The model under review builds one solid part; all positions refer to its coordinate system, in mm. Face numbers are marked on the shaded views. A direction names the side the tool comes from. Give positions to 0.01 mm unless a question says otherwise; leave off trailing zeros. Loops run counter-clockwise (first coordinate to the right, second up) from the corner with the lowest first, then second, coordinate; pieces in that order, holes last. Notation, with made-up numbers: (-16, 59) -> (-12, 59) arc R16 ccw to (-12, 78) -> close; hole circle Ø10 at (42.25, 31). An arc over 180 degrees is marked (long way). Write each question's results on one line, items separated by ' | '. Start each with the question number.
Q1. We need section D-D (x = -2.5). Write out the cut boundary in (y, z), plus the area to 3 significant figures.
Q2. Wall thickness on L1, parallel to X at y = -40.5, z = 3.75; L2, parallel to X at y = -39, z = 4.25; L3, parallel to Y at x = 0, z = 3.5: over which ranges is each line inside the solid? List them lowest first. Write a range as [from, to].
Q3. We need section B-B (x = 34.5). Write out the cut boundary in (y, z), plus the area to 3 significant figures.
Q4. We need section C-C (y = 0). Write out the cut boundary in (x, z).
Q5. Machinability: for the marked faces 1 and 2, which of the approach directions +Z, -Z, +X, -X, +Y, -Y give a long, thin tool a straight path to every point of the face, cutting with its end or side? Answer none if there is none.
Q6. Insertion check: pin 1 Ø1.5 at (y, z) = (-27, 3.5) entering from +X. The pin has a flat end and moves straight along its axis. Give the tip position at first contact, or say it passes through.
Q7. We need section A-A (z = 2.25). Give the number of separate pieces and of enclosed holes in the cut face, plus the area to 3 significant figures.
Q8. Mouldability with a two-part tool opening along Y and no side actions: class the marked faces 3, 4 and 5 as released by +Y, released by -Y, zero draft, split by the parting line, or undercut.
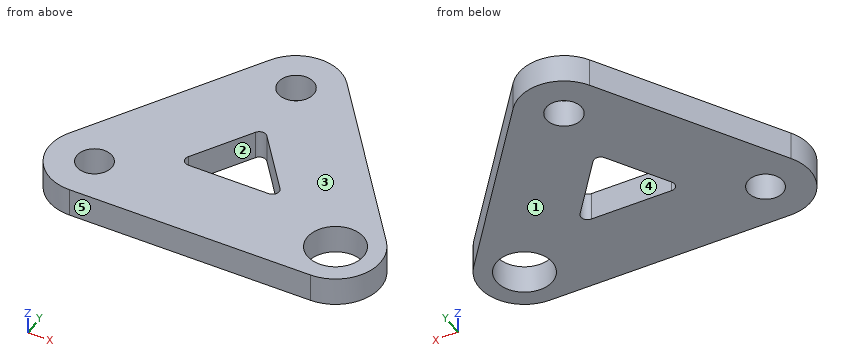
from build123d import *

# Parameters (mm, degrees)
SKETCH1_R           = 10
SKETCH1_R_2         = 3.875
SKETCH1_R_3         = 3.9375
SKETCH1_R_4         = 6.223
BOSS_EXTRUDE1_DEPTH = 6.35
FILLET1_R           = 1.5


with BuildPart() as part:
    # Sketch1 → Boss-Extrude1 (new body)
    # profile 1 of 4: a face of its own
    with BuildSketch(Plane.XY):
        with BuildLine():
            Line((-8.593850937, 5.113289165), (-31.697797638, -33.717269329))
            ThreePointArc((-31.697797638, -33.717269329), (-20.452391437, -29.188501934), (-13.103946701, -38.830558493))
            ThreePointArc((-13.103946701, -38.830558493), (-16.032878889, -45.901626305), (-23.103946701, -48.830558493))
            Line((-23.103946701, -48.830558493), (30.579912659, -48.830558493))
            ThreePointArc((30.579912659, -48.830558493), (21.583526758, -34.464205241), (38.436192426, -32.643566638))
            Line((38.436192426, -32.643566638), (7.856279768, 6.186991855))
            ThreePointArc((7.856279768, 6.186991855), (9.44888347, 3.273927483), (10, 0))
            ThreePointArc((10, 0), (-2.651555264, -9.642056559), (-8.593850937, 5.113289165))
        make_face()
        Polygon((-9.254840748, -30.955558493), (0.905857228, -13.878581033), (14.354349844, -30.955558493), align=None, mode=Mode.SUBTRACT)
    # profile 2 of 4: a face of its own
    with BuildSketch(Plane.XY):
        with Locations((-23.103946701, -38.830558493)):
            Circle(SKETCH1_R)
        with Locations((-23.103946701, -38.830558493)):
            Circle(SKETCH1_R_2, mode=Mode.SUBTRACT)
    # profile 3 of 4: a face of its own
    with BuildSketch(Plane.XY):
        Circle(SKETCH1_R)
        Circle(SKETCH1_R_3, mode=Mode.SUBTRACT)
    # profile 4 of 4: a face of its own
    with BuildSketch(Plane.XY):
        with Locations((30.579912659, -38.830558493)):
            Circle(SKETCH1_R)
        with Locations((30.579912659, -38.830558493)):
            Circle(SKETCH1_R_4, mode=Mode.SUBTRACT)
    extrude(amount=BOSS_EXTRUDE1_DEPTH)

    # Fillet1
    fillet1_edges = [part.edges().sort_by_distance(p)[0] for p in [
        (0.905857228, -13.878581033, 3.175),
        (-9.254840748, -30.955558493, 3.175),
        (14.354349844, -30.955558493, 3.175),
    ]]
    fillet(fillet1_edges, radius=FILLET1_R)


solid = part.part
Output:
1) outline: (-48.83, 0) -> (-30.96, 0) -> (-30.96, 6.35) -> (-48.83, 6.35) -> close; (-19.6, 0) -> (-3.04, 0) -> (-3.04, 6.35) -> (-19.6, 6.35) -> close; (3.04, 0) -> (9.68, 0) -> (9.68, 6.35) -> (3.04, 6.35) -> close | area: 261 mm2
2) L1: [-32.96, -26.6], [-19.61, 24.59], [36.57, 40.44] | L2: [-33.1, -26.98], [-19.23, 24.36], [36.8, 40.58] | L3: [-48.83, -30.96], [-15.48, -3.94], [3.94, 10]
3) outline: (-48.03, 0) -> (-43.66, 0) -> (-43.66, 6.35) -> (-48.03, 6.35) -> close; (-34, 0) -> (-27.65, 0) -> (-27.65, 6.35) -> (-34, 6.35) -> close | area: 68.1 mm2
4) outline: (-11.64, 0) -> (-3.94, 0) -> (-3.94, 6.35) -> (-11.64, 6.35) -> close; (3.94, 0) -> (12.73, 0) -> (12.73, 6.35) -> (3.94, 6.35) -> close
5) face 1: -Z, +X, -X, +Y, -Y | face 2: +Z, -Z
6) pin 1: x = 34.58
7) separate pieces: 1 | enclosed holes: 4 | area: 2,430 mm2
8) face 3: zero draft | face 4: undercut | face 5: released by -Y
